Check sheet for the modelled part. Datum: model origin and axes. Units: mm. A direction names the side the tool comes from. Round coordinates to 2 decimals unless told otherwise and drop trailing zeros. Order: outer loops, then holes, each group sorted by start corner. A loop starts at its lowest first (then second) coordinate and runs counter-clockwise, first axis right, second up.
Q1. Scan lines: probe 1 along Z at (x, y) = (14, 5.5); probe 2 along X at (y, z) = (1.75, 18); probe 3 along X at (y, z) = (4.5, 13.75). Record each from-to range of solid material in increasing order.
Q2. Set-up check for faces 1 (the flat face through (-16, 8, 13)), 2 (the flat face through (16, 8, 13)), 3 (the flat face through (16, 0, 13)): record each of +Z, -Z, +X, -X, +Y, -Y from which the full face is reachable in a straight line by a thin tool's end or side.
Q3. Cross-section at D-D on x = 0. Record the cut outline in (y, z), then the cut area to 3 significant figures.
Q4. Cross-section at A-A on z = 6. Record the cut outline in (x, y), then the cut area to 3 significant figures.
Q5. Depth check by flat-ended pin: P1, Ø3, axis at x = -15.56, z = 6, coming from the -Y side; P2, Ø6.5, axis at x = 15, z = 11.5, coming from the +Y side; P3, Ø4, axis at y = 11, z = 19.5, coming from the -X side; P4, Ø12, axis at x = -2.5, z = 9.5, coming from the -Y side. Enter the tip coordinate at first touch or a pass-through.
Q6. Cross-section at C-C on z = 20.5. Record the cut outline in (x, y).
Q7. Mould release check, pull along X, two halves, no side actions. Record for faces 4 (the flat face through (0, 18, 13)), 5 (the cylindrical face through (17.13, 4.06, 6.65)), 6 (the flat face through (-12.56, 11, 14)), 7 (the flat face through (18.56, 4, 13)): +X half, -X half, draft (parallel to the pull), parting line (faces both ways), or undercut.
Q8. Cross-section at B-B on y = 3. Record the cut outline in (x, z).
from build123d import *

# Parameters (mm, degrees)
BOSS_EXTRU_1_DEPTH      = 27
ESQUISSE5_R             = 1.7
ENL_V_MAT_EXTRU_1_DEPTH = 18
ESQUISSE6_W             = 6
ESQUISSE6_H             = 27
ENL_V_MAT_EXTRU_2_DEPTH = 10
CONG_1_R                = 5


with BuildPart() as part:
    # Esquisse1 → Boss.-Extru.1 (new body)
    with BuildSketch(Plane.XY):
        with BuildLine():
            Line((-12.560062385, 0), (-18.560062385, 0))
            Line((-18.560062385, 0), (-18.560062385, 18))
            Line((-18.560062385, 18), (18.560062385, 18))
            Line((18.560062385, 18), (18.560062385, 0))
            Line((18.560062385, 0), (12.560062385, 0))
            ThreePointArc((12.560062385, 0), (0, 12.560062385), (-12.560062385, 0))
        make_face()
    extrude(amount=BOSS_EXTRU_1_DEPTH)

    # Esquisse5 → Enlèv. mat.-Extru.1 (cut)
    with BuildSketch(Plane(origin=(0, 18, 0), x_dir=(1, 0, 0), z_dir=(0, 1, 0))):
        with Locations((15.560062385, -6)):
            Circle(ESQUISSE5_R)
        with Locations((15.560062385, -18)):
            Circle(ESQUISSE5_R)
        with Locations((-15.560062385, -6)):
            Circle(ESQUISSE5_R)
        with Locations((-15.560062385, -18)):
            Circle(ESQUISSE5_R)
    extrude(amount=-ENL_V_MAT_EXTRU_1_DEPTH, mode=Mode.SUBTRACT)

    # Esquisse6 → Enlèv. mat.-Extru.2 (cut)
    with BuildSketch(Plane(origin=(0, 18, 0), x_dir=(1, 0, 0), z_dir=(0, 1, 0))):
        with Locations((15.560062385, -13.5)):
            Rectangle(ESQUISSE6_W, ESQUISSE6_H)
        with Locations((-15.560062385, -13.5)):
            Rectangle(ESQUISSE6_W, ESQUISSE6_H)
    extrude(amount=-ENL_V_MAT_EXTRU_2_DEPTH, mode=Mode.SUBTRACT)

    # Congé1
    cong_1_edges = [part.edges().sort_by_distance(p)[0] for p in [
        (12.560062385, 18, 13.5),
        (-12.560062385, 18, 13.5),
    ]]
    fillet(cong_1_edges, radius=CONG_1_R)


solid = part.part
Results found:
1. probe 1: z = 0 to 5.32, 6.68 to 17.32, 18.68 to 27
1. probe 2: x = -18.56 to -17.26, -13.86 to -12.44, 12.44 to 13.86, 17.26 to 18.56
1. probe 3: x = -18.56 to -11.73, 11.73 to 18.56
2. face 1: +Z, -Z, -X, +Y
2. face 2: +Z, -Z, +X, +Y
2. face 3: +Z, -Z, +X, -X, -Y
3. outline: (12.56, 0) - (18, 0) - (18, 27) - (12.56, 27) - close
3. area: 147 mm2
4. outline: (-18.56, 0) - (-17.26, 0) - (-17.26, 8) - (-18.56, 8) - close; (-13.86, 0) - (-12.56, 0) arc R12.56 cw to (12.56, 0) - (13.86, 0) - (13.86, 8) - (12.56, 8) - (12.56, 13) arc R5 ccw to (7.56, 18) - (-7.56, 18) arc R5 ccw to (-12.56, 13) - (-12.56, 8) - (-13.86, 8) - close; (17.26, 0) - (18.56, 0) - (18.56, 8) - (17.26, 8) - close
4. area: 235 mm2
5. P1: passes through
5. P2: stops at y = 15.73
5. P3: stops at x = -12.56
5. P4: stops at y = 9.25
6. outline: (-18.56, 0) - (-12.56, 0) arc R12.56 cw to (12.56, 0) - (18.56, 0) - (18.56, 8) - (12.56, 8) - (12.56, 13) arc R5 ccw to (7.56, 18) - (-7.56, 18) arc R5 ccw to (-12.56, 13) - (-12.56, 8) - (-18.56, 8) - close
7. face 4: draft
7. face 5: undercut
7. face 6: -X half
7. face 7: +X half
8. outline: (-18.56, 0) - (-12.2, 0) - (-12.2, 27) - (-18.56, 27) - close; (12.2, 0) - (18.56, 0) - (18.56, 27) - (12.2, 27) - close; hole circle Ø3.4 at (-15.56, 6); hole circle Ø3.4 at (-15.56, 18); hole circle Ø3.4 at (15.56, 6); hole circle Ø3.4 at (15.56, 18)
